Could you check a few things on this model? Use its own coordinates, in mm. A direction names the side the tool comes from. Round coordinates to 2 decimals unless told otherwise and drop trailing zeros. Write each loop counter-clockwise with the first axis right and the second up, starting at its lowest first coordinate (ties: lowest second). Pieces come first, ordered by that corner, then holes. Notation, with made-up numbers: (2.5, 84.5) -> (40.5, 84.5) arc R18 ccw to (40.5, 115.5) -> close; hole circle Ø2 at (-10.75, 68). An arc over 180 degrees is marked (long way). Answer as CSV lines item,"result". Start each with the question number.
Q1. Imagine slicing it at A-A on x = 0. Please give me the cut outline in (y, z), and give its area (3 significant figures).
Q2. Will this pin go through, and if not, where does the flat tip stop? pin 1 Ø1 at (x, z) = (4, 2) entering from -Y.
Q3. Imagine slicing it at C-C on z = 2.6. Please give me the cut outline in (x, y), and give its area (3 significant figures).
Q4. For faces 1 (the flat face through (-5.2, -1, -1)), 2 (the conical face through (-0.675, 2.142, 1.609)), which set-ups out of +Z, -Z, +X, -X, +Y, -Y let a thin tool reach every point of the face, with its end or its side?
Q5. Imagine slicing it at B-B on y = 0. Please give me the cut outline in (x, z).
Q6. If I drill on line 1 (Z direction, x = -2, y = 3.25); line 2 (Z direction, x = 3.75, y = 3.25); line 3 (Z direction, x = 3, y = 1.25), over which ranges is the centre line in solid material (lowest first)? Write a range as [from, to].
Q7. Imagine slicing it at D-D on z = 1.7. Please give me the cut outline in (x, y).
from build123d import *

# Parameters (mm, degrees)
SKETCH001_W    = 10.4
SKETCH001_H    = 9.76
PAD_DEPTH      = 0.75
PAD_DEPTH_BACK = 3


with BuildPart() as opening_revolve:
    # Sketch006 → Revolution (revolve)
    with BuildSketch(Plane.YZ):
        with BuildLine():
            Line((0, 0.49), (2.75, 0.49))
            ThreePointArc((2.75, 0.49), (3.188748, 1.229792), (2.329167, 1.26))
            Line((2.329167, 1.26), (2.129167, 1.26))
            Line((2.129167, 1.26), (2.129167, 1.51))
            Line((2.129167, 1.51), (4, 3.09))
            Line((4, 3.09), (0, 3.09))
            Line((0, 3.09), (0, 0.49))
        make_face()
    revolve(axis=Axis((0, 0, 0), (0, 0, 1)))


with BuildPart() as fusion:
    # Sketch001 → Pad (new body, two sides)
    with BuildSketch(Plane.XY) as pad_sk:
        with Locations((0, -0.48)):
            Rectangle(SKETCH001_W, SKETCH001_H)
    extrude(amount=PAD_DEPTH)
    extrude(pad_sk.sketch, amount=-PAD_DEPTH_BACK)


with BuildPart() as fusion_1:
    # Body001 placement: moved
    add(fusion.part.moved(Location((0, 0, 0.483))))

    # Fusion: union opening_revolve
    add(opening_revolve.part)


solid = fusion_1.part
Checks:
1,outline,"(-5.36, -2.52) -> (4.4, -2.52) -> (4.4, 1.23) -> (3.19, 1.23) arc R0.5 ccw to (2.33, 1.26) -> (2.13, 1.26) -> (2.13, 1.51) -> (4, 3.09) -> (-4, 3.09) -> (-2.13, 1.51) -> (-2.13, 1.26) -> (-2.33, 1.26) arc R0.5 ccw to (-3.19, 1.23) -> (-5.36, 1.23) -> close"
1,area,"47.8 mm^2"
2,pin 1,"through"
3,outline,"circle Ø6.84 at (0, 0)"
3,area,"36.7 mm^2"
4,face 1,"+Z, -Z, -X, +Y, -Y"
4,face 2,"none"
5,outline,"(-5.2, -2.52) -> (5.2, -2.52) -> (5.2, 1.23) -> (3.19, 1.23) arc R0.5 ccw to (2.33, 1.26) -> (2.13, 1.26) -> (2.13, 1.51) -> (4, 3.09) -> (-4, 3.09) -> (-2.13, 1.51) -> (-2.13, 1.26) -> (-2.33, 1.26) arc R0.5 ccw to (-3.19, 1.23) -> (-5.2, 1.23) -> close"
6,line 1,"[-2.52, 1.23], [2.93, 3.09]"
6,line 2,"[-2.52, 1.23]"
6,line 3,"[-2.52, 1.23], [2.46, 3.09]"
7,outline,"circle Ø4.71 at (0, 0)"
